from build123d import *

# Parameters (mm, degrees)
BOSS_EXTRUDE1_DEPTH = 170.18
FILLET1_R           = 3.175
SKETCH2_R           = 3.175
CUT_EXTRUDE1_DEPTH  = 174.929734088
SKETCH3_R           = 3.175
CUT_EXTRUDE2_DEPTH  = 174.929734088
SKETCH4_R           = 3.175
CUT_EXTRUDE3_DEPTH  = 174.494504308
SKETCH5_R           = 3.175
CUT_EXTRUDE4_DEPTH  = 174.494504308


with BuildPart() as part:
    # Sketch1 → Boss-Extrude1 (new body)
    with BuildSketch(Plane(origin=(0, 0, 0), x_dir=(1, 0, 0), z_dir=(0, 1, 0))):
        Polygon((0, 0), (3.175, 0), (3.175, -22.225), (25.4, -22.225), (25.4, -25.4), (0, -25.4), align=None)
    extrude(amount=BOSS_EXTRUDE1_DEPTH)

    # Fillet1
    fillet1_edges = [part.edges().sort_by_distance(p)[0] for p in [
        (3.175, 85.09, 22.225),
    ]]
    fillet(fillet1_edges, radius=FILLET1_R)

    # Sketch2 → Cut-Extrude1 (cut, through all)
    with BuildSketch(Plane.ZY):
        with Locations((9.652, 160.528)):
            Circle(SKETCH2_R)
    extrude(amount=-CUT_EXTRUDE1_DEPTH, mode=Mode.SUBTRACT)

    # Sketch3 → Cut-Extrude2 (cut, through all)
    with BuildSketch(Plane.ZY):
        with Locations((9.652, 9.652)):
            Circle(SKETCH3_R)
    extrude(amount=-CUT_EXTRUDE2_DEPTH, mode=Mode.SUBTRACT)

    # Sketch4 → Cut-Extrude3 (cut, through all)
    with BuildSketch(Plane(origin=(0, 0, 22.225), x_dir=(-1, 0, 0), z_dir=(0, 0, -1))):
        with Locations((-15.748, 9.652)):
            Circle(SKETCH4_R)
    extrude(amount=-CUT_EXTRUDE3_DEPTH, mode=Mode.SUBTRACT)

    # Sketch5 → Cut-Extrude4 (cut, through all)
    with BuildSketch(Plane(origin=(0, 0, 22.225), x_dir=(-1, 0, 0), z_dir=(0, 0, -1))):
        with Locations((-15.875, 160.655)):
            Circle(SKETCH5_R)
    extrude(amount=-CUT_EXTRUDE4_DEPTH, mode=Mode.SUBTRACT)


solid = part.part
Here's how the part is built. I have some questions about the finished solid (model axes, mm). A direction names the side the tool comes from. Give positions to 0.01 mm unless a question says otherwise; leave off trailing zeros. Order: outer loops, then holes, each group sorted by start corner. A loop starts at its lowest first (then second) coordinate and runs counter-clockwise, first axis right, second up. Notation, with made-up numbers: M -39.75,37 L 19.25,37 A16 ccw 19.25,52 Z; hole C 27,69.25 d8. An arc over 180 degrees is marked long. Answer as a JSON object with one key per item and string values. Group by question number.
1) Suppose I cut it at C-C, the plane y = 45. Write out the boundary of the cut face in (x, z) (3 decimals).
2) We'd pull the mould along Y, two halves only. Please class faces 3 (the cylindrical face through (16.563, 157.556, 23.79)), 4 (the flat face through (7, 0, 23)), 5 (the flat face through (0, 84, 13)): pulls with the +Y half, pulls with the -Y half, needs draft (parallel to the pull), parting line crosses it, or undercut.
3) Suppose I cut it at D-D, the plane z = 2.25. Write out the boundary of the cut face in (x, y) (3 decimals), plus the area to 3 significant figures.
4) Suppose I cut it at A-A, the plane x = 14.75. Write out the boundary of the cut face in (y, z) (3 decimals).
5) I'm going to push flat-ended pins straight in: pin 1 Ø1 at (x, y) = (15, 144) entering from -Z (3 decimals); pin 2 Ø12 at (x, z) = (5.5, 8) entering from +Y; pin 3 Ø8 at (y, z) = (45.5, 8) entering from +X (3 decimals); pin 4 Ø2 at (x, y) = (6, 95.5) entering from -Z. Where does each tip first touch, or does it pass through?
6) On a 3-axis mill with a long thin cutter (end or side, diameter ignored), from which of +Z, -Z, +X, -X, +Y, -Y can I reach the whole of each face in a straight line? I mean faces 1 (the cylindrical face through (1.57, 9.79, 6.48)), 2 (the flat face through (3.175, 84, 9)). Say none if no direction works.
7) Suppose I cut it at B-B, the plane z = 11. Write out the boundary of the cut face in (x, y) (3 decimals).
8) Please list where these lines run through material, in increasing order: L1, parallel to X at y = 47, z = 7.5 (3 decimals); L2, parallel to Y at x = 13.75, z = 23; L3, parallel to Z at x = 17.5, y = 66 (3 decimals). Write a range as [from, to].
Results found:
{
 "1": {"outline": "M 0,0 L 3.175,0 L 3.175,19.05 A3.175 cw 6.35,22.225 L 25.4,22.225 L 25.4,25.4 L 0,25.4 Z"},
 "2": {"face 3": "undercut", "face 4": "pulls with the -Y half", "face 5": "needs draft"},
 "3": {"outline": "M 0,0 L 3.175,0 L 3.175,170.18 L 0,170.18 Z", "area": "540 mm²"},
 "4": {"outline": "M 0,22.225 L 6.638,22.225 L 6.638,25.4 L 0,25.4 Z; M 12.666,22.225 L 157.686,22.225 L 157.686,25.4 L 12.666,25.4 Z; M 163.624,22.225 L 170.18,22.225 L 170.18,25.4 L 163.624,25.4 Z"},
 "5": {"pin 1": "z = 22.225", "pin 2": "y = 170.18", "pin 3": "x = 3.175", "pin 4": "z = 21.92"},
 "6": {"face 1": "+X, -X", "face 2": "-Z, +X, +Y, -Y"},
 "7": {"outline": "M 0,0 L 3.175,0 L 3.175,6.777 L 0,6.777 Z; M 0,12.527 L 3.175,12.527 L 3.175,157.653 L 0,157.653 Z; M 0,163.403 L 3.175,163.403 L 3.175,170.18 L 0,170.18 Z"},
 "8": {"L1": "[0, 3.175]", "L2": "[0, 7.18], [12.12, 158.3], [163.01, 170.18]", "L3": "[22.225, 25.4]"}
}
